Build history of the part. All positions in model axes, mm. Round coordinates to 2 decimals unless told otherwise and drop trailing zeros. Write each loop counter-clockwise with the first axis right and the second up, starting at its lowest first coordinate (ties: lowest second). Pieces come first, ordered by that corner, then holes.
from build123d import *

# Parameters (mm, degrees)
SKETCH1_W                    = 127
SKETCH1_H                    = 76.2
BOSS_EXTRUDE1_DEPTH          = 3.175
SKETCH2_R                    = 9.84885
SKETCH2_R_2                  = 14.2875
CUT_EXTRUDE1_DEPTH           = 75.324844433
CHAMFER1_SIZE                = 19.05
F_10_0_1935_DIAMETER_HOLE1_D = 4.9149
FILLET1_R                    = 3.175


with BuildPart() as part:
    # Sketch1 → Boss-Extrude1 (new, symmetric)
    with BuildSketch(Plane.XY):
        Rectangle(SKETCH1_W, SKETCH1_H)
    extrude(amount=BOSS_EXTRUDE1_DEPTH, both=True)

    # Sketch2 → Cut-Extrude1 (cut, through all)
    with BuildSketch(Plane.XY.offset(3.175)):
        with Locations((-51.92522, 0)):
            Circle(SKETCH2_R)
        with Locations((38.1, 0)):
            Circle(SKETCH2_R_2)
    extrude(amount=-CUT_EXTRUDE1_DEPTH, mode=Mode.SUBTRACT)

    # Chamfer1
    chamfer1_edges = [part.edges().sort_by_distance(p)[0] for p in [
        (63.5, -38.1, 0),
        (63.5, 38.1, 0),
    ]]
    chamfer(chamfer1_edges, length=CHAMFER1_SIZE)

    # #10 (0.1935) Diameter Hole1 (through all)
    with Locations(Plane.XY.offset(3.175)):
        with Locations((-51.92522, 25.4), (-51.92522, -25.4), (38.1, 25.4), (38.1, -25.4), (-51.92522, 0), (38.1, 0)):
            Hole(F_10_0_1935_DIAMETER_HOLE1_D / 2)

    # Fillet1
    fillet1_edges = [part.edges().sort_by_distance(p)[0] for p in [
        (44.45, 38.1, 0),
        (63.5, -19.05, 0),
        (63.5, 19.05, 0),
        (44.45, -38.1, 0),
    ]]
    fillet(fillet1_edges, radius=FILLET1_R)


solid = part.part
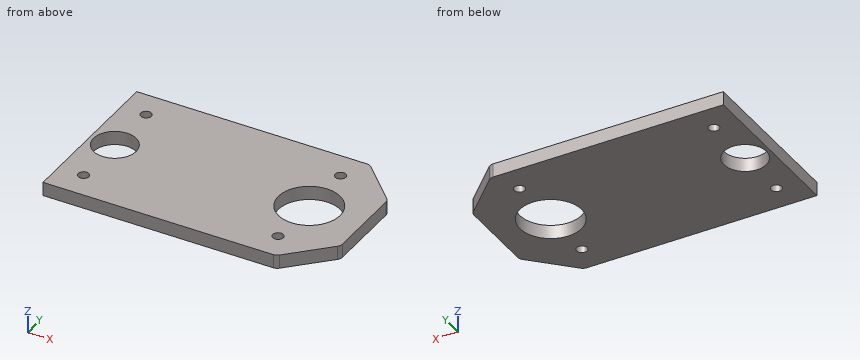
1) Slice it at D-D (y = 25.4). Write the cut outline in (x, z) (3 decimals).
Results:
outline: (-63.5, -3.175) - (-54.383, -3.175) - (-54.383, 3.175) - (-63.5, 3.175) - close; (-49.468, -3.175) - (35.643, -3.175) - (35.643, 3.175) - (-49.468, 3.175) - close; (40.557, -3.175) - (57.15, -3.175) - (57.15, 3.175) - (40.557, 3.175) - close
2) Wall check: L1, parallel to Y at x = -52, z = -2; L2, parallel to Y at x = 38.1, z = -1; L3, parallel to X at y = 9, z = 1.75. Give the ranges that are in metal, low to high.
Results:
L1: y = -38.1 to -27.86, -22.94 to -9.85, 9.85 to 22.94, 27.86 to 38.1
L2: y = -38.1 to -27.86, -22.94 to -14.29, 14.29 to 22.94, 27.86 to 38.1
L3: x = -63.5 to -55.93, -47.93 to 27, 49.2 to 63.5
3) Pin check, flat tips, straight feed: pin 1 Ø3 at (x, y) = (38.1, 25.4) entering from +Z; pin 2 Ø5.5 at (x, y) = (38.1, -25.4) entering from +Z (3 decimals). Stop position of each tip, or through.
Results:
pin 1: passes through
pin 2: stops at z = 3.175
4) Slice it at A-A (y = 0). Write the cut outline in (x, z) (1 decimal).
Results:
outline: (-63.5, -3.2) - (-61.8, -3.2) - (-61.8, 3.2) - (-63.5, 3.2) - close; (-42.1, -3.2) - (23.8, -3.2) - (23.8, 3.2) - (-42.1, 3.2) - close; (52.4, -3.2) - (63.5, -3.2) - (63.5, 3.2) - (52.4, 3.2) - close
5) Slice it at C-C (z = -1.5). Count the separate pieces of the cut face and the enclosed holes in it, plus the area to 3 significant figures.
Results:
separate pieces: 1
enclosed holes: 6
area: 8,290 mm2
6) Slice it at B-B (x = 38.1). Write the cut outline in (y, z) (1 decimal), plus the area to 3 significant figures.
Results:
outline: (-38.1, -3.2) - (-27.9, -3.2) - (-27.9, 3.2) - (-38.1, 3.2) - close; (-22.9, -3.2) - (-14.3, -3.2) - (-14.3, 3.2) - (-22.9, 3.2) - close; (14.3, -3.2) - (22.9, -3.2) - (22.9, 3.2) - (14.3, 3.2) - close; (27.9, -3.2) - (38.1, -3.2) - (38.1, 3.2) - (27.9, 3.2) - close
area: 240 mm2
